Autodesk Inventor part; units mm, degrees
ref_plane "YZ Plane" through (0, 0, 0) normal (1, 0, 0) x (0, 1, 0)
ref_plane "XZ Plane" through (0, 0, 0) normal (0, 1, 0) x (-1, 0, 0)
ref_plane "XY Plane" through (0, 0, 0) normal (0, 0, 1) x (1, 0, 0)
sketch "Sketch1" plane through (0, 0, 0) normal (0, 0, 1) x (1, 0, 0)
  line L0 (0, 0) -> (0, 700)
  line L1 (0, 0) -> (2000, 0)
  line L2 (0, 700) -> (2000, 700)
  line L3 (2000, 700) -> (2000, 0)
  line L4 (2000, 0) -> (0, 0)
  line L5 (0, 0) -> (0, 700)
  dimension "d0" = 700
  dimension "d1" = 2000
extrude "Extrusion1" add sketch "Sketch1" along normal blind 1500
sketch "Sketch2" plane through (0, 700, 0) normal (0, 1, 0) x (1, 0, 0)
  line L0 (1974.1538, -1477.007) -> (20.8481, -1477.007)
  line L1 (20.8481, -1477.007) -> (20.8481, -20.8481)
  line L2 (20.8481, -20.8481) -> (1974.1538, -20.8481)
  line L3 (1974.1538, -20.8481) -> (1974.1538, -1477.007)
  point P0 (0, 0)
extrude "Extrusion2" cut sketch "Sketch2" against normal blind 692.25
sketch "Sketch3" plane through (0, 7.75, 0) normal (0, 1, 0) x (1, 0, 0)
  line L0 (1974.1538, -20.8481) -> (1974.1538, -1477.007)
  line L1 (20.8481, -20.8481) -> (1974.1538, -20.8481)
  line L2 (1974.1538, -1477.007) -> (20.8481, -20.8481)
  line L3 (1974.1538, -1477.007) -> (20.8481, -1477.007)
  line L4 (20.8481, -1477.007) -> (1974.1538, -20.8481)
  line L5 (997.5009, -748.9276) -> (997.5009, -1112.664)
  circle A0 centre (997.5009, -1112.664) radius 140.4471
  line L6 (997.5009, -1253.1111) -> (997.5009, -1303.1111)
  circle A1 centre (997.5009, -1303.1111) radius 25
  circle A2 centre (832.5689, -1207.8876) radius 25
  circle A3 centre (832.5689, -1017.4404) radius 25
  circle A4 centre (997.5009, -922.2169) radius 25
  circle A5 centre (1162.433, -1017.4404) radius 25
  circle A6 centre (1162.433, -1207.8876) radius 25
  circle A7 centre (997.5009, -1112.664) radius 226.7645
  circle A8 centre (997.5009, -1112.664) radius 226.7645
  point P0 (0, 0)
  dimension "d9" = 50
  dimension "d11" = 50
  dimension "d14" = 360
extrude "Extrusion3" add sketch "Sketch3" along normal blind 112.25 contours A7
properties part number "Robot Volume and wall" material "Wood (Birch)"
Geometry: final body of the model. Coordinates: model frame, mm. A direction names the side the tool comes from. Give positions to 0.01 mm unless a question says otherwise; leave off trailing zeros. Write each loop counter-clockwise with the first axis right and the second up, starting at its lowest first coordinate (ties: lowest second). Pieces come first, ordered by that corner, then holes.
1. Section query A-A, the plane x = 237. Return loops of the section in (y, z), then the cut area to 3 significant figures.
2. Reachability of faces 4 (the flat face through (2000, 355, 740)), 5 (the flat face through (996, 7.75, 1111)) from +Z, -Z, +X, -X, +Y, -Y: full face, straight path, thin tool, end or side. Return the list, or none.
3. Draft query along X for faces 1 (the flat face through (0, 345, 740)), 2 (the flat face through (986, 355, 0)), 3 (the flat face through (1162, 7.75, 1208)). Return one class per face: released by +X, released by -X, zero draft, split by the parting line, or undercut.
4. Section query B-B, the plane y = 237.5. Return loops of the section in (x, z), then the cut area to 3 significant figures.
5. Section query C-C, the plane z = 686. Return loops of the section in (x, y), then the cut area to 3 significant figures.
6. Line query: probe 1 along X at (y, z) = (336, 374.5); probe 2 along Z at (x, y) = (390.5, 34.5); probe 3 along Y at (x, z) = (668, 559.5). Output: solid intervals per line, ascending.
7. Pin query (flat end, axial travel): P1, Ø15, axis at x = 829.5, z = 1014.5, coming from the +Y side; P2, Ø25, axis at x = 820.5, z = 1201, coming from the +Y side. Return the tip coordinate at first contact, or that it passes through.
8. Section query D-D, the plane x = 924. Return loops of the section in (y, z).
Computed:
1. outline: (0, 0) - (700, 0) - (700, 20.85) - (7.75, 20.85) - (7.75, 1477.01) - (700, 1477.01) - (700, 1500) - (0, 1500) - close
1. area: 42,000 mm2
2. face 4: +Z, -Z, +X, +Y, -Y
2. face 5: +Y
3. face 1: released by -X
3. face 2: zero draft
3. face 3: undercut
4. outline: (0, 0) - (2000, 0) - (2000, 1500) - (0, 1500) - close; hole (20.85, 20.85) - (1974.15, 20.85) - (1974.15, 1477.01) - (20.85, 1477.01) - close
4. area: 156,000 mm2
5. outline: (0, 0) - (2000, 0) - (2000, 700) - (1974.15, 700) - (1974.15, 7.75) - (20.85, 7.75) - (20.85, 700) - (0, 700) - close
5. area: 47,800 mm2
6. probe 1: x = 0 to 20.85, 1974.15 to 2000
6. probe 2: z = 0 to 20.85, 1477.01 to 1500
6. probe 3: y = 0 to 7.75
7. P1: stops at y = 7.75
7. P2: stops at y = 120
8. outline: (0, 0) - (700, 0) - (700, 20.85) - (7.75, 20.85) - (7.75, 898.14) - (120, 898.14) - (120, 992.99) - (7.75, 992.99) - (7.75, 1232.34) - (120, 1232.34) - (120, 1327.19) - (7.75, 1327.19) - (7.75, 1477.01) - (700, 1477.01) - (700, 1500) - (0, 1500) - close
